from build123d import *

# Parameters (mm, degrees)
BOSS_EXTRUDE1_DEPTH = 0.35


with BuildPart() as part:
    # Sketch1 → Revolve1 (revolve)
    with BuildSketch(Plane.XY):
        with BuildLine():
            Line((0, 0), (5.4, 0))
            Line((5.4, 0), (5.4, 2))
            Line((5.4, 2), (5, 2))
            Line((5, 2), (5, 8.65))
            ThreePointArc((5, 8.65), (3.535533906, 12.185533906), (0, 13.65))
            Line((0, 13.65), (0, 0))
        make_face()
    revolve(axis=Axis((0, 0, 0), (0, 1, 0)))

    # Sketch3 → Boss-Extrude1 (add, symmetric)
    with BuildSketch(Plane.XY):
        Polygon((1.54, -3), (1.54, 0), (3.54, 0), (3.54, -3), (2.94, -3), (2.94, -20), (2.14, -20), (2.14, -3), align=None)
        Polygon((-2.14, -17), (-2.94, -17), (-2.94, -3), (-3.54, -3), (-3.54, 0), (-1.54, 0), (-1.54, -3), (-2.14, -3), align=None)
    extrude(amount=BOSS_EXTRUDE1_DEPTH, both=True)


solid = part.part
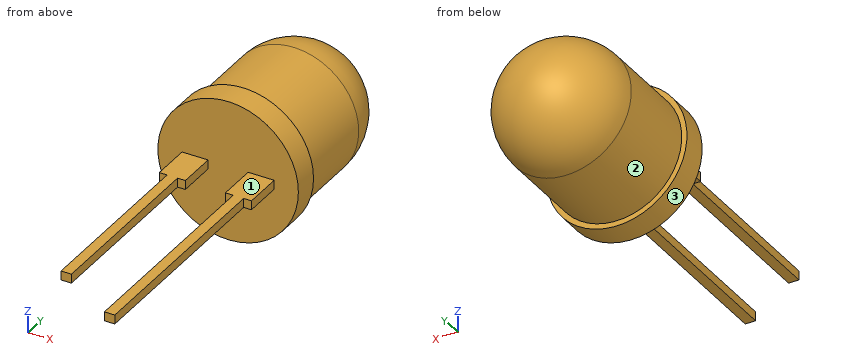
CAD build for the part. Positions are in the model's coordinates, mm. Face numbers are marked on the shaded views. A direction names the side the tool comes from. Round coordinates to 2 decimals unless told otherwise and drop trailing zeros. Order: outer loops, then holes, each group sorted by start corner. A loop starts at its lowest first (then second) coordinate and runs counter-clockwise, first axis right, second up. Notation, with made-up numbers: (31.5, 76) - (39.5, 76) arc R15 ccw to (39.5, 80) - close; hole circle Ø3 at (-15, -19.75). An arc over 180 degrees is marked (long way). Return JSON: item names as keys, results as strings.
(1) Cut at B-B (x = 0). Give the cut face in (y, z).
Answer key:
{"outline": "(0, -5.4) - (2, -5.4) - (2, -5) - (8.65, -5) arc R5 ccw to (8.65, 5) - (2, 5) - (2, 5.4) - (0, 5.4) - close"}
(2) Pin check, flat tips, straight feed: pin 1 Ø2 at (x, y) = (3, -10) entering from -Z; pin 2 Ø0.8 at (y, z) = (-7.5, 0) entering from +X; pin 3 Ø4 at (x, z) = (-0.5, -1) entering from -Y. Stop position of each tip, or through.
Answer key:
{"pin 1": "stops at z = -0.35", "pin 2": "stops at x = 2.94", "pin 3": "stops at y = -17"}
(3) Wall check: probe 1 along X at (y, z) = (-4, -0.25); probe 2 along Y at (x, z) = (-2.5, 4.5); probe 3 along Z at (x, y) = (2.5, -8.5). Give the ranges that are in metal, low to high. Write a range as from..to.
Answer key:
{"probe 1": "x = -2.94..-2.14, 2.14..2.94", "probe 2": "y = 0..2", "probe 3": "z = -0.35..0.35"}
(4) Tool access for the marked faces 1, 2 and 3: list every direction of +Z, -Z, +X, -X, +Y, -Y with a clear straight run to the whole face (end or side of a thin tool).
Answer key:
{"face 1": "+Z, +X, -X, -Y", "face 2": "+Y", "face 3": "+Y, -Y"}
(5) Cut at C-C (z = 0). Give the cut face in (x, y), then the cut area to 3 significant figures.
Answer key:
{"outline": "(-5.4, 0) - (-3.54, 0) - (-3.54, -3) - (-2.94, -3) - (-2.94, -17) - (-2.14, -17) - (-2.14, -3) - (-1.54, -3) - (-1.54, 0) - (1.54, 0) - (1.54, -3) - (2.14, -3) - (2.14, -20) - (2.94, -20) - (2.94, -3) - (3.54, -3) - (3.54, 0) - (5.4, 0) - (5.4, 2) - (5, 2) - (5, 8.65) arc R5 ccw to (-5, 8.65) - (-5, 2) - (-5.4, 2) - close", "area": "164 mm^2"}
(6) Cut at D-D (y = -1). Give the cut face in (x, z).
Answer key:
{"outline": "(-3.54, -0.35) - (-1.54, -0.35) - (-1.54, 0.35) - (-3.54, 0.35) - close; (1.54, -0.35) - (3.54, -0.35) - (3.54, 0.35) - (1.54, 0.35) - close"}
(7) Cut at A-A (y = -9). Give the cut face in (x, z), then the cut area to 3 significant figures.
Answer key:
{"outline": "(-2.94, -0.35) - (-2.14, -0.35) - (-2.14, 0.35) - (-2.94, 0.35) - close; (2.14, -0.35) - (2.94, -0.35) - (2.94, 0.35) - (2.14, 0.35) - close", "area": "1.12 mm^2"}
